Part model, mm, in its own coordinate system. A direction names the side the tool comes from. Give positions to 0.01 mm unless a question says otherwise; leave off trailing zeros. Write each loop counter-clockwise with the first axis right and the second up, starting at its lowest first coordinate (ties: lowest second). Pieces come first, ordered by that corner, then holes. Notation, with made-up numbers: M 35.25,46.5 L 54.25,46.5 A24 cw 54.25,79.5 Z; hole C 75,48.25 d5. An arc over 180 degrees is marked long. Use a Markdown table: item, result.
```python
from build123d import *

# Parameters (mm, degrees)
PAD_DEPTH       = 30
SKETCH002_R     = 8
POCKET_DEPTH    = 30
SKETCH003_R     = 8
PAD001_DEPTH    = 25
SKETCH004_R     = 8
POCKET001_DEPTH = 5
PAD002_DEPTH    = 17.5
POCKET002_DEPTH = 12.5


with BuildPart() as part:
    # Sketch → Pad (new body)
    with BuildSketch(Plane.XZ):
        Polygon((-15, -14.95402), (15, -14.95402), (15, -7.95402), (32, -7.95402), (32, -2.95402), (23, 5.04598), (13, 5.04598), (13, 20.04598), (-13, 20.04598), (-13, 5.04598), (-23, 5.04598), (-32, -2.95402), (-32, -7.95402), (-15, -7.95402), align=None)
    extrude(amount=PAD_DEPTH)

    # Sketch002 (on Face16 of Pad) → Pocket (cut)
    with BuildSketch(Plane.XZ.offset(30)):
        with Locations((0, 20.04598)):
            Circle(SKETCH002_R)
    extrude(amount=-POCKET_DEPTH, mode=Mode.SUBTRACT)

    # Sketch003 (on Face5 of Pocket) → Pad001 (join)
    with BuildSketch(Plane.XZ.offset(30)):
        with Locations((0, 20.04598)):
            Circle(SKETCH003_R)
    extrude(amount=-PAD001_DEPTH)

    # Sketch004 (on Face20 of Pad001) → Pocket001 (cut)
    with BuildSketch(Plane.XZ.offset(30)):
        with Locations((0, 20.04598)):
            Circle(SKETCH004_R)
    extrude(amount=-POCKET001_DEPTH, mode=Mode.SUBTRACT)

    # Sketch005 (on Face5 of Pocket001) → Pad002 (join)
    with BuildSketch(Plane.XZ.offset(30)):
        Polygon((-23, 5.04598), (-13, 5.04598), (-13, 20.04598), (-16, 20.04598), align=None)
        Polygon((23, 5.04598), (13, 5.04598), (13, 20.04598), (16, 20.04598), align=None)
    extrude(amount=-PAD002_DEPTH)

    # Sketch006 (on Face24 of Pad002) → Pocket002 (cut)
    with BuildSketch(Plane.XZ.offset(30)):
        Polygon((-23, 5.04598), (-16, 20.04598), (-13, 20.04598), (-13, 5.04598), align=None)
        Polygon((23, 5.04598), (16, 20.04598), (13, 20.04598), (13, 5.04598), align=None)
    extrude(amount=-POCKET002_DEPTH, mode=Mode.SUBTRACT)


solid = part.part
```
1. Cut at A-A, the plane y = -23.5. Give the cut face in (x, z), then the cut area to 3 significant figures.
Findings below:
| item | result |
|---|---|
| outline | M -32,-7.95 L -15,-7.95 L -15,-14.95 L 15,-14.95 L 15,-7.95 L 32,-7.95 L 32,-2.95 L 23,5.05 L 13,5.05 L 13,20.05 L 8,20.05 A8 ccw -8,20.05 L -13,20.05 L -13,5.05 L -23,5.05 L -32,-2.95 Z |
| area | 1,460 mm2 |
2. Cut at C-C, the plane z = 19. Give the cut face in (x, y), then the cut area to 3 significant figures.
Findings below:
| item | result |
|---|---|
| outline | M -16.49,-17.5 L -13,-17.5 L -13,-30 L -7.93,-30 L -7.93,-25 L 7.93,-25 L 7.93,-30 L 13,-30 L 13,-17.5 L 16.49,-17.5 L 16.49,-12.5 L 13,-12.5 L 13,0 L 7.93,0 L 7.93,-5 L -7.93,-5 L -7.93,0 L -13,0 L -13,-12.5 L -16.49,-12.5 Z |
| area | 656 mm2 |
3. Tool access for faces 4 (the flat face through (11, -15, 20.046)), 5 (the flat face through (-24, -15, -7.954)), 6 (the flat face through (-17, -17.5, 11)), 7 (the flat face through (18, -6, 5.046)), 8 (the flat face through (-13, -6, 13)): list every direction of +Z, -Z, +X, -X, +Y, -Y with a clear straight run to the whole face (end or side of a thin tool).
Findings below:
| item | result |
|---|---|
| face 4 | +Z, +X, +Y, -Y |
| face 5 | -Z, -X, +Y, -Y |
| face 6 | +Z, -X, -Y |
| face 7 | +Z, +X, +Y |
| face 8 | +Z, -X, +Y |
4. Drill centre lines: L1, parallel to Z at x = -23, y = -19; L2, parallel to X at y = -5, z = -11; L3, parallel to X at y = -22.25, z = 8. Where is each one in solid material? Low to high.
Findings below:
| item | result |
|---|---|
| L1 | -7.95 to 5.05 |
| L2 | -15 to 15 |
| L3 | -13 to 13 |
5. Cut at D-D, the plane y = -27.5. Give the cut face in (x, z).
Findings below:
| item | result |
|---|---|
| outline | M -32,-7.95 L -15,-7.95 L -15,-14.95 L 15,-14.95 L 15,-7.95 L 32,-7.95 L 32,-2.95 L 23,5.05 L 13,5.05 L 13,20.05 L 8,20.05 A8 cw -8,20.05 L -13,20.05 L -13,5.05 L -23,5.05 L -32,-2.95 Z |
6. Drop flat-ended pins along their axis: P1, Ø6.5, axis at x = 10.5, y = -9, coming from the +Z side; P2, Ø5, axis at x = -18.5, y = -6, coming from the +Z side; P3, Ø14, axis at y = -4.5, z = 15, coming from the -X side. Give the stop position or say it passes through.
Findings below:
| item | result |
|---|---|
| P1 | z = 23.43 |
| P2 | z = 5.05 |
| P3 | x = -13 |
7. Two-plate mould, pull along X, no slides. Class faces 1 (the cylindrical face through (-0.18, -2.54, 12.05)), 2 (the flat face through (-18, -6, 5.046)), 3 (the flat face through (27.56, -14.79, 0.99)): released by +X, released by -X, zero draft, split by the parting line, or undercut.
Findings below:
| item | result |
|---|---|
| face 1 | undercut |
| face 2 | zero draft |
| face 3 | released by +X |
8. Cut at B-B, the plane x = 0. Give the cut face in (y, z).
Findings below:
| item | result |
|---|---|
| outline | M -30,-14.95 L 0,-14.95 L 0,12.05 L -5,12.05 L -5,28.05 L -25,28.05 L -25,12.05 L -30,12.05 Z |
